Input: dimensioned drawing with shaded views. Units: mm. Origin: part minimum x, y, z. Give positions to 0.01 mm unless a question says otherwise; leave off trailing zeros. Write each loop counter-clockwise with the first axis right and the second up, starting at its lowest first coordinate (ties: lowest second). Pieces come first, ordered by that corner, then holes. Notation, with made-up numbers: M 24.25,35 L 42.25,35 A13 cw 42.25,54 Z; hole C 32.5,-15.5 d7. An arc over 180 degrees is marked long. Answer as a JSON object with one key per item and string values.
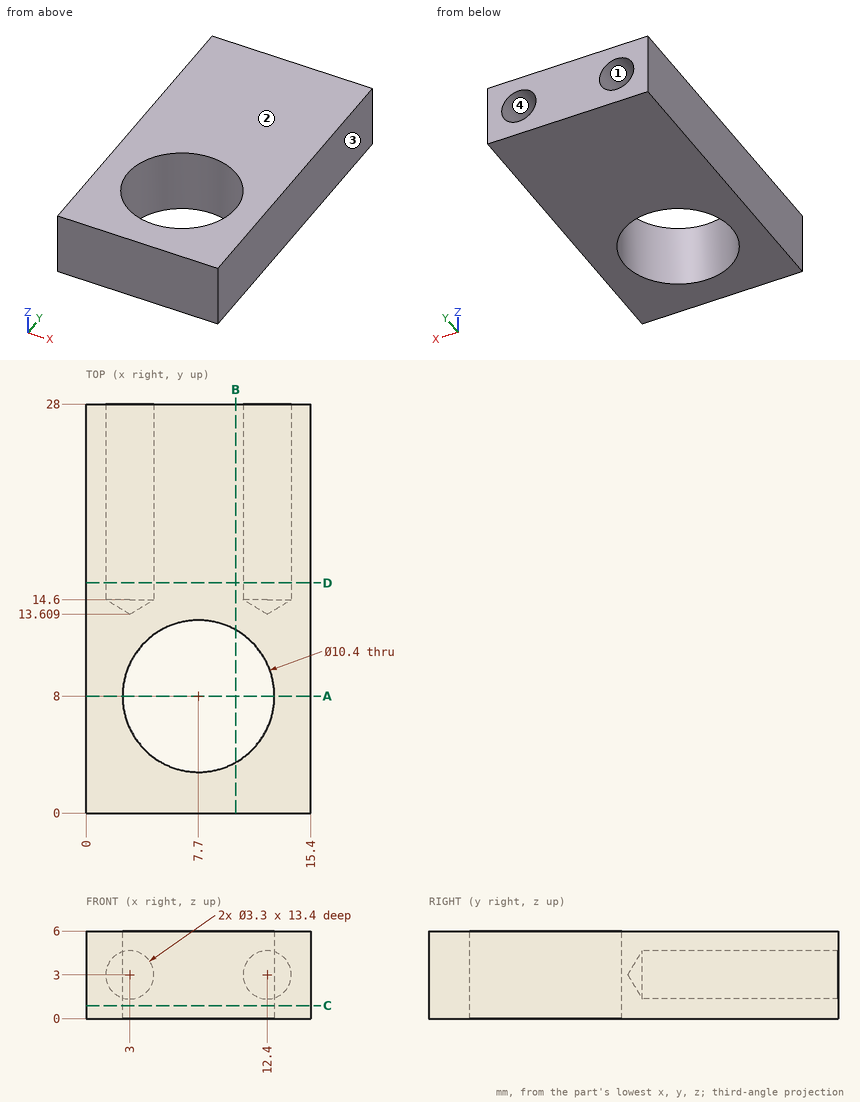
1) Cut plane B-B on x = 10.25. Return loops of the section in (y, z).
Geometry check:
{"outline": "M 0,0 L 3.47,0 L 3.47,6 L 0,6 Z; M 12.53,0 L 28,0 L 28,6 L 12.53,6 Z"}
2) Contact query for flat-ended pins moving along their axis: P1, Ø5, axis at x = 5.5, y = 14.5, coming from the -Z side; P2, Ø2.5, axis at x = 3, z = 3, coming from the +Y side. Output: stop coordinate, or through.
Geometry check:
{"P1": "stops at z = 0", "P2": "stops at y = 14.36"}
3) Line query: line 1 (X direction, y = 23, z = 3); line 2 (Z direction, x = 12.4, y = 20.25); line 3 (X direction, y = 26.5, z = 4.1). Output: solid intervals per line, ascending. Write a range as from..to.
Geometry check:
{"line 1": "x = 0..1.35, 4.65..10.75, 14.05..15.4", "line 2": "z = 0..1.35, 4.65..6", "line 3": "x = 0..1.77, 4.23..11.17, 13.63..15.4"}
4) Pull-direction query (Z, two-part tool) for the marked faces 1, 2, 3 and 4; classes: pulls with the +Z half, pulls with the -Z half, needs draft (parallel to the pull), parting line crosses it, or undercut.
Geometry check:
{"face 1": "undercut", "face 2": "pulls with the +Z half", "face 3": "needs draft", "face 4": "undercut"}
5) Cut plane D-D on y = 15.75. Return loops of the section in (x, z).
Geometry check:
{"outline": "M 0,0 L 15.4,0 L 15.4,6 L 0,6 Z; hole C 3,3 d3.3; hole C 12.4,3 d3.3"}
6) Cut plane A-A on y = 8. Return loops of the section in (x, z).
Geometry check:
{"outline": "M 0,0 L 2.5,0 L 2.5,6 L 0,6 Z; M 12.9,0 L 15.4,0 L 15.4,6 L 12.9,6 Z"}
7) Cut plane C-C on z = 0.9. Return loops of the section in (x, y).
Geometry check:
{"outline": "M 0,0 L 15.4,0 L 15.4,28 L 0,28 Z; hole C 7.7,8 d10.4"}
